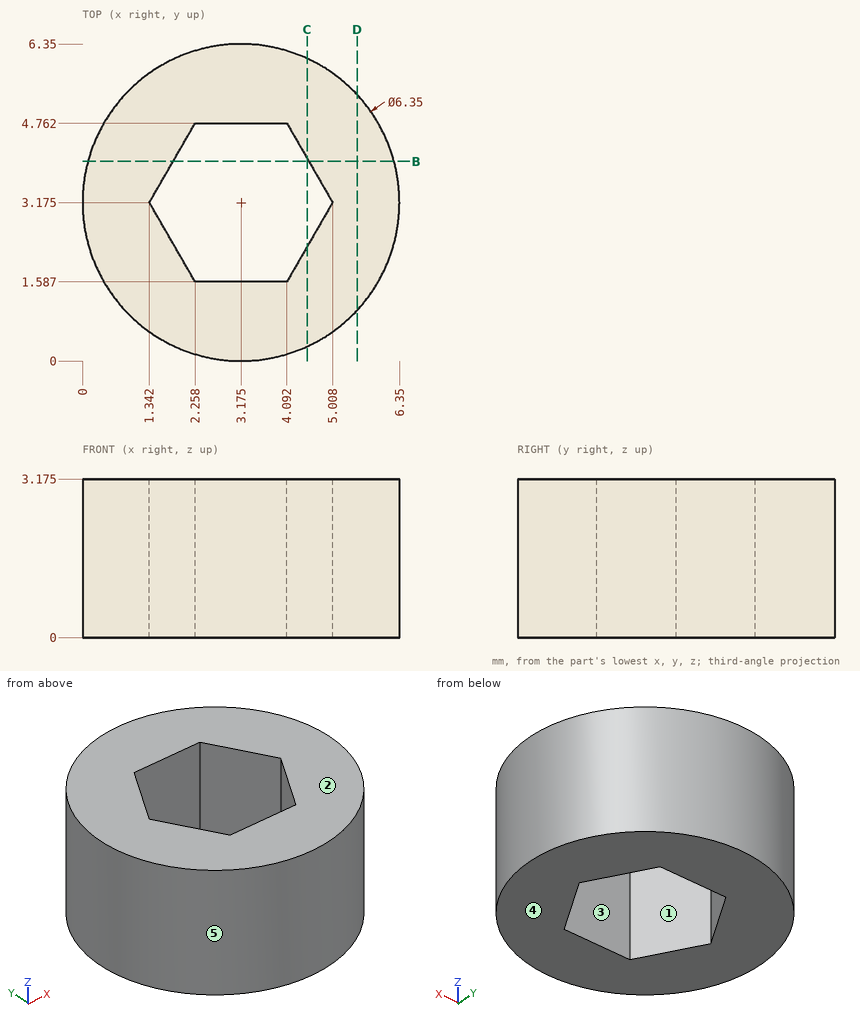
Geometry check sheet. Reference: drawing and pictorial views, mm from the part's lowest x, y, z. A direction names the side the tool comes from. Round coordinates to 2 decimals unless told otherwise and drop trailing zeros. Write each loop counter-clockwise with the first axis right and the second up, starting at its lowest first coordinate (ties: lowest second). Pieces come first, ordered by that corner, then holes. Notation, with made-up numbers: (-6.75, -32) -> (15.25, -32) arc R20 ccw to (15.25, -6) -> close; hole circle Ø10 at (22.5, -25). An arc over 180 degrees is marked (long way). Put each result on its own line as item: value.
1) Cross-section at C-C, the plane x = 4.5. Enter the section's corners in (y, z) (1 decimal).
Recorded:
outline: (0.3, 0) -> (2.3, 0) -> (2.3, 3.2) -> (0.3, 3.2) -> close; (4.1, 0) -> (6.1, 0) -> (6.1, 3.2) -> (4.1, 3.2) -> close
2) Access from +Z, -Z, +X, -X, +Y, -Y to the whole of each face (thin tool, end or side, straight path). Record for the marked faces 1 and 2.
Recorded:
face 1: +Z, -Z
face 2: +Z, +X, -X, +Y, -Y
3) Thickness scan on probe 1 along Y at (x, z) = (2.75, 1.8); probe 2 along X at (y, z) = (2, 0.9) (1 decimal); probe 3 along Y at (x, z) = (4, 0.8). Record the ranges inside material, lowest first. Write a range as from..to.
Recorded:
probe 1: y = 0.03..1.59, 4.76..6.32
probe 2: x = 0.2..2, 4.3..6.1
probe 3: y = 0.11..1.59, 4.76..6.24
4) Depth check by flat-ended pin: P1, Ø1.5, axis at x = 3, z = 1.5, coming from the -Y side. Enter the tip coordinate at first touch or a pass-through.
Recorded:
P1: stops at y = 0
5) Release check for a two-part mould opening along Y. For the marked faces 3, 4 and 5 record: pulls with the +Y half, pulls with the -Y half, needs draft (parallel to the pull), parting line crosses it, or undercut.
Recorded:
face 3: undercut
face 4: needs draft
face 5: parting line crosses it
6) Cross-section at B-B, the plane y = 4. Enter the section's corners in (x, z) (1 decimal).
Recorded:
outline: (0.1, 0) -> (1.8, 0) -> (1.8, 3.2) -> (0.1, 3.2) -> close; (4.5, 0) -> (6.2, 0) -> (6.2, 3.2) -> (4.5, 3.2) -> close
7) Cross-section at D-D, the plane x = 5.5. Enter the section's corners in (y, z) (1 decimal), plus the area to 3 significant figures.
Recorded:
outline: (1, 0) -> (5.3, 0) -> (5.3, 3.2) -> (1, 3.2) -> close
area: 13.7 mm2
